```python
from build123d import *

# Parameters (mm, degrees)
SKETCH2_W                     = 59
SKETCH2_H                     = 25
BOSS_EXTRUDE1_DEPTH           = 1.5875
EDGE_FLANGE2_STRIP_W          = 9.525
EDGE_FLANGE2_STRIP_H          = 1.5875
EDGE_FLANGE2_STRIP_CUT_DEPTH  = 9.5
EDGE_FLANGE2_RELIEF_W         = 10.31875
EDGE_FLANGE2_RELIEF_H         = 0.79375
EDGE_FLANGE2_RELIEF_CUT_DEPTH = 1.5875
EDGE_FLANGE2_DEPTH            = 9.5
EDGE_FLANGE3_STRIP_W          = 9.525
EDGE_FLANGE3_STRIP_H          = 1.5875
EDGE_FLANGE3_STRIP_CUT_DEPTH  = 9.5
EDGE_FLANGE3_RELIEF_W         = 10.31875
EDGE_FLANGE3_RELIEF_H         = 0.79375
EDGE_FLANGE3_RELIEF_CUT_DEPTH = 1.5875
EDGE_FLANGE3_DEPTH            = 9.5
CUT_EXTRUDE1_REACH            = 69.127
SKETCH16_R                    = 1
SKETCH18_W                    = 38.4125
SKETCH18_H                    = 12
BOSS_EXTRUDE2_DEPTH           = 1.5875
SKETCH19_R                    = 1.5
SKETCH19_W                    = 9.5
SKETCH19_H                    = 3.825
CUT_EXTRUDE2_DEPTH            = 1.5875
EDGE_FLANGE4_STRIP_W          = 9.525
EDGE_FLANGE4_STRIP_H          = 1.5875
EDGE_FLANGE4_STRIP_CUT_DEPTH  = 40
EDGE_FLANGE4_DEPTH            = 40
FILLET1_R                     = 2


# Sheet-metal steps are written as plain solids
with BuildPart() as part:
    # Sketch2 → Boss-Extrude1 (new body)
    with BuildSketch(Plane(origin=(0, 0, 0), x_dir=(1, 0, 0), z_dir=(0, 1, 0))):
        with Locations((29.5, 12.5)):
            Rectangle(SKETCH2_W, SKETCH2_H)
    extrude(amount=BOSS_EXTRUDE1_DEPTH)

    # Edge-Flange2 strip (across the edge) → Edge-Flange2 strip cut (cut)
    with BuildSketch(Plane(origin=(59, 1.5875, -25), x_dir=(0, 0, 1), z_dir=(-1, 0, 0))):
        with Locations((-1.5875, -0.79375)):
            Rectangle(EDGE_FLANGE2_STRIP_W, EDGE_FLANGE2_STRIP_H)
    extrude(amount=EDGE_FLANGE2_STRIP_CUT_DEPTH, mode=Mode.SUBTRACT)

    # Edge-Flange2 relief (on the sheet) → Edge-Flange2 relief cut (cut)
    with BuildSketch(Plane(origin=(59, 1.5875, -21.825), x_dir=(0, 0, 1), z_dir=(0, 1, 0))):
        with Locations((-4.365625, -9.896875)):
            Rectangle(EDGE_FLANGE2_RELIEF_W, EDGE_FLANGE2_RELIEF_H)
    extrude(amount=-EDGE_FLANGE2_RELIEF_CUT_DEPTH, mode=Mode.SUBTRACT)

    # Edge-Flange2 section (across the edge) → Edge-Flange2 (add)
    with BuildSketch(Plane(origin=(59, 1.5875, -25), x_dir=(0, 0, 1), z_dir=(-1, 0, 0))):
        with BuildLine():
            Line((0, 1.5875), (0, 18.4125))
            Line((0, 18.4125), (1.5875, 18.4125))
            Line((1.5875, 18.4125), (1.5875, 1.5875))
            ThreePointArc((1.5875, 1.5875), (2.052467985, 0.464967985), (3.175, 0))
            Line((3.175, 0), (3.175, -1.5875))
            ThreePointArc((3.175, -1.5875), (0.92993597, -0.65756403), (0, 1.5875))
        make_face()
    extrude(amount=EDGE_FLANGE2_DEPTH)

    # Edge-Flange3 strip (across the edge) → Edge-Flange3 strip cut (cut)
    with BuildSketch(Plane(origin=(9.5, 1.5875, -25), x_dir=(0, 0, 1), z_dir=(-1, 0, 0))):
        with Locations((-1.5875, -0.79375)):
            Rectangle(EDGE_FLANGE3_STRIP_W, EDGE_FLANGE3_STRIP_H)
    extrude(amount=EDGE_FLANGE3_STRIP_CUT_DEPTH, mode=Mode.SUBTRACT)

    # Edge-Flange3 relief (on the sheet) → Edge-Flange3 relief cut (cut)
    with BuildSketch(Plane(origin=(9.5, 1.5875, -21.825), x_dir=(0, 0, 1), z_dir=(0, 1, 0))):
        with Locations((-4.365625, 0.396875)):
            Rectangle(EDGE_FLANGE3_RELIEF_W, EDGE_FLANGE3_RELIEF_H)
    extrude(amount=-EDGE_FLANGE3_RELIEF_CUT_DEPTH, mode=Mode.SUBTRACT)

    # Edge-Flange3 section (across the edge) → Edge-Flange3 (add)
    with BuildSketch(Plane(origin=(9.5, 1.5875, -25), x_dir=(0, 0, 1), z_dir=(-1, 0, 0))):
        with BuildLine():
            Line((0, 1.5875), (0, 18.4125))
            Line((0, 18.4125), (1.5875, 18.4125))
            Line((1.5875, 18.4125), (1.5875, 1.5875))
            ThreePointArc((1.5875, 1.5875), (2.052467985, 0.464967985), (3.175, 0))
            Line((3.175, 0), (3.175, -1.5875))
            ThreePointArc((3.175, -1.5875), (0.92993597, -0.65756403), (0, 1.5875))
        make_face()
    extrude(amount=EDGE_FLANGE3_DEPTH)

    # Sketch16 → Cut-Extrude1 (cut, up to next)
    with BuildSketch(Plane(origin=(0, 0, -25), x_dir=(-1, 0, 0), z_dir=(0, 0, -1)), mode=Mode.PRIVATE) as cut_extrude1_sk1:
        with Locations(Location((-54.25, 16.5875, 0), (0, 0, 90))):
            Circle(SKETCH16_R)
    cut_extrude1_tool1 = extrude(cut_extrude1_sk1.sketch, amount=-CUT_EXTRUDE1_REACH, mode=Mode.PRIVATE) & part.part
    # Sketch16 → Cut-Extrude1 (cut, up to next)
    with BuildSketch(Plane(origin=(0, 0, -25), x_dir=(-1, 0, 0), z_dir=(0, 0, -1)), mode=Mode.PRIVATE) as cut_extrude1_sk2:
        with Locations(Location((-54.25, 6.5875, 0), (0, 0, 90))):
            Circle(SKETCH16_R)
    cut_extrude1_tool2 = extrude(cut_extrude1_sk2.sketch, amount=-CUT_EXTRUDE1_REACH, mode=Mode.PRIVATE) & part.part
    # Sketch16 → Cut-Extrude1 (cut, up to next)
    with BuildSketch(Plane(origin=(0, 0, -25), x_dir=(-1, 0, 0), z_dir=(0, 0, -1)), mode=Mode.PRIVATE) as cut_extrude1_sk3:
        with Locations(Location((-4.75, 6.5875, 0), (0, 0, 270))):
            Circle(SKETCH16_R)
    cut_extrude1_tool3 = extrude(cut_extrude1_sk3.sketch, amount=-CUT_EXTRUDE1_REACH, mode=Mode.PRIVATE) & part.part
    # Sketch16 → Cut-Extrude1 (cut, up to next)
    with BuildSketch(Plane(origin=(0, 0, -25), x_dir=(-1, 0, 0), z_dir=(0, 0, -1)), mode=Mode.PRIVATE) as cut_extrude1_sk4:
        with Locations(Location((-4.75, 16.5875, 0), (0, 0, 270))):
            Circle(SKETCH16_R)
    cut_extrude1_tool4 = extrude(cut_extrude1_sk4.sketch, amount=-CUT_EXTRUDE1_REACH, mode=Mode.PRIVATE) & part.part
    add(cut_extrude1_tool1.solids().sort_by_distance((54.25, 16.5875, -25))[0], mode=Mode.SUBTRACT)
    add(cut_extrude1_tool2.solids().sort_by_distance((54.25, 6.5875, -25))[0], mode=Mode.SUBTRACT)
    add(cut_extrude1_tool3.solids().sort_by_distance((4.75, 6.5875, -25))[0], mode=Mode.SUBTRACT)
    add(cut_extrude1_tool4.solids().sort_by_distance((4.75, 16.5875, -25))[0], mode=Mode.SUBTRACT)

    # Sketch18 → Boss-Extrude2 (add)
    with BuildSketch(Plane(origin=(0, 1.5875, 0), x_dir=(1, 0, 0), z_dir=(0, 1, 0))):
        with Locations((29.5, 31)):
            Rectangle(SKETCH18_W, SKETCH18_H)
    extrude(amount=-BOSS_EXTRUDE2_DEPTH)

    # Sketch19 → Cut-Extrude2 (cut)
    with BuildSketch(Plane(origin=(0, 1.5875, 0), x_dir=(1, 0, 0), z_dir=(0, 1, 0))):
        with Locations(Location((4.75, 17.825, 0), (0, 0, 270))):
            Circle(SKETCH19_R)
        with Locations(Location((4.75, 7.825, 0), (0, 0, 270))):
            Circle(SKETCH19_R)
        with Locations(Location((54.25, 17.825, 0), (0, 0, 90))):
            Circle(SKETCH19_R)
        with Locations(Location((54.25, 7.825, 0), (0, 0, 90))):
            Circle(SKETCH19_R)
        with Locations((54.25, 1.9125)):
            Rectangle(SKETCH19_W, SKETCH19_H)
        with Locations((4.75, 1.9125)):
            Rectangle(SKETCH19_W, SKETCH19_H)
    extrude(amount=-CUT_EXTRUDE2_DEPTH, mode=Mode.SUBTRACT)

    # Edge-Flange4 strip (across the edge) → Edge-Flange4 strip cut (cut)
    with BuildSketch(Plane(origin=(9.5, 1.5875, 0), x_dir=(0, 0, -1), z_dir=(1, 0, 0))):
        with Locations((-3.175, -0.79375)):
            Rectangle(EDGE_FLANGE4_STRIP_W, EDGE_FLANGE4_STRIP_H)
    extrude(amount=EDGE_FLANGE4_STRIP_CUT_DEPTH, mode=Mode.SUBTRACT)

    # Edge-Flange4 section (across the edge) → Edge-Flange4 (add)
    with BuildSketch(Plane(origin=(9.5, 1.5875, 0), x_dir=(0, 0, -1), z_dir=(1, 0, 0))):
        with BuildLine():
            Line((-1.5875, 1.5875), (-1.5875, 18.4125))
            Line((-1.5875, 18.4125), (0, 18.4125))
            Line((0, 18.4125), (0, 1.5875))
            ThreePointArc((0, 1.5875), (0.464967985, 0.464967985), (1.5875, 0))
            Line((1.5875, 0), (1.5875, -1.5875))
            ThreePointArc((1.5875, -1.5875), (-0.65756403, -0.65756403), (-1.5875, 1.5875))
        make_face()
    extrude(amount=EDGE_FLANGE4_DEPTH)

    # Fillet1
    fillet1_edges = [part.edges().sort_by_distance(p)[0] for p in [
        (10.29375, 0.79375, -37),
        (48.70625, 0.79375, -37),
        (0, 0.79375, -3.825),
        (59, 0.79375, -3.825),
        (9.5, 20, 0.79375),
        (49.5, 20, 0.79375),
        (59, 20, -24.20625),
        (49.5, 20, -24.20625),
        (9.5, 20, -24.20625),
        (0, 20, -24.20625),
    ]]
    fillet(fillet1_edges, radius=FILLET1_R)


solid = part.part
```
Here's how the part is built. I have some questions about the finished solid (model axes, mm). A direction names the side the tool comes from. Give positions to 0.01 mm unless a question says otherwise; leave off trailing zeros. Order: outer loops, then holes, each group sorted by start corner. A loop starts at its lowest first (then second) coordinate and runs counter-clockwise, first axis right, second up. Notation, with made-up numbers: M -35,5 L -30,5 A24 ccw -30,44 Z; hole C 53,-32.5 d7. An arc over 180 degrees is marked long. Use a Markdown table: item, result. Add a question column.
1. For pin 1 Ø5 at (x, y) = (4.5, 13) entering from +Z; pin 2 Ø0.5 at (y, z) = (0.5, -30) entering from +X; pin 3 Ø4 at (x, y) = (10, 8.5) entering from -Z, each with a flat end and sliding along its axis, tell me the tip position at first contact or that it passes through.
2. If we mould it in two halves opening along X, with no side actions, what happens to faces 1 (the flat face through (48.706, 1, -28)), 2 (the flat face through (9.5, 9, -24)), 3 (the cylindrical face through (10.895, 0.783, -36.43)), 4 (the flat face through (5, 12, -23.412))? For each: +X half, -X half, draft (parallel to the pull), parting line (faces both ways), or undercut.
3. I need wall thicknesses on probe 1 along Y at (x, z) = (4.75, -24.2); probe 2 along Y at (x, z) = (4.75, -24.05); probe 3 along X at (y, z) = (14.25, -24). Which ranges of each line are inside material? Lowest first, please. Write a range as from..to.
4. Suppose I cut it at A-A (y = 14). List the corners of the cut face in (x, z) for me.
5. Suppose I cut it at B-B (x = 54.25). Give the number of separate pieces and of enclosed holes in the cut face, and give its area (3 significant figures).
6. On a 3-axis mill with a long thin cutter (end or side, diameter ignored), from which of +Z, -Z, +X, -X, +Y, -Y can I reach the whole of each face in a straight line? I mean faces 5 (the cylindrical face through (55.714, 0.805, -17.5)), 6 (the flat face through (9.5, 7, 1)), 7 (the flat face through (29, 12, 0)), 8 (the flat face through (29, 1, -37)), 9 (the flat face through (49.5, 9, -24)). Say none if no direction works.
7. Suppose I cut it at C-C (y = 6.25). List the corners of the cut face in (x, z) for me, and give its area (3 significant figures).
Results list:
| question | item | result |
|---|---|---|
| 1 | pin 1 | stops at z = -23.41 |
| 1 | pin 2 | stops at x = 48.71 |
| 1 | pin 3 | stops at z = -25 |
| 2 | face 1 | undercut |
| 2 | face 2 | undercut |
| 2 | face 3 | -X half |
| 2 | face 4 | draft |
| 3 | probe 1 | y = 1.07..5.59, 7.59..15.59, 17.59..20 |
| 3 | probe 2 | y = 0.91..5.59, 7.59..15.59, 17.59..20 |
| 3 | probe 3 | x = 0..9.5, 49.5..59 |
| 4 | outline | M 0,-25 L 9.5,-25 L 9.5,-23.41 L 0,-23.41 Z; M 9.5,0 L 49.5,0 L 49.5,1.59 L 9.5,1.59 Z; M 49.5,-25 L 59,-25 L 59,-23.41 L 49.5,-23.41 Z |
| 5 | separate pieces | 5 |
| 5 | enclosed holes | 0 |
| 5 | area | 45.3 mm² |
| 6 | face 5 | +Y, -Y |
| 6 | face 6 | +Z, -X, +Y, -Y |
| 6 | face 7 | -Z, +X, -X, +Y |
| 6 | face 8 | -Z, +X, -X, +Y, -Y |
| 6 | face 9 | -Z, +Y, -Y |
| 7 | outline | M 0,-25 L 3.81,-25 L 3.81,-23.41 L 0,-23.41 Z; M 5.69,-25 L 9.5,-25 L 9.5,-23.41 L 5.69,-23.41 Z; M 9.5,0 L 49.5,0 L 49.5,1.59 L 9.5,1.59 Z; M 49.5,-25 L 53.31,-25 L 53.31,-23.41 L 49.5,-23.41 Z; M 55.19,-25 L 59,-25 L 59,-23.41 L 55.19,-23.41 Z |
| 7 | area | 87.7 mm² |
